Autodesk Inventor part; units mm, degrees
ref_plane "YZ Plane" through (0, 0, 0) normal (1, 0, 0) x (0, 1, 0)
ref_plane "XZ Plane" through (0, 0, 0) normal (0, 1, 0) x (-1, 0, 0)
ref_plane "XY Plane" through (0, 0, 0) normal (0, 0, 1) x (1, 0, 0)
sketch "Sketch1" plane through (0, 0, 0) normal (0, 0, 1) x (1, 0, 0)
  line L0 (100.1576, -44) -> (109, -35.1576)
  line L1 (109, -35.1576) -> (109, 35)
  line L2 (109, 35) -> (41.05, 35)
  line L3 (41.05, 35) -> (28, 30)
  line L4 (28, 30) -> (-28, 30)
  line L5 (-28, 30) -> (-30, 28)
  line L6 (-30, 28) -> (-30, -28)
  line L7 (-30, -28) -> (-28, -30)
  line L8 (-28, -30) -> (28, -30)
  line L9 (28, -30) -> (90.0667, -30)
  line L10 (90.0667, -30) -> (90.0667, -44)
  line L11 (90.0667, -44) -> (100.1576, -44)
  circle A0 centre (101, -8.23) radius 1.6
  circle A1 centre (101, 1.77) radius 1.6
  circle A2 centre (101, 29.77) radius 1.6
  circle A3 centre (85, 29.77) radius 1.6
  circle A4 centre (85, 1.77) radius 1.6
  circle A5 centre (85, -8.23) radius 1.6
  circle A6 centre (64.15, 11.27) radius 1.6
  circle A7 centre (47.85, 11.27) radius 1.6
  circle A8 centre (25, 0) radius 1.95
  circle A9 centre (0, 25) radius 1.95
  circle A10 centre (-25, -25) radius 1.95
  circle A11 centre (25, 25) radius 1.95
  circle A12 centre (-25, 25) radius 1.95
  circle A13 centre (25, -25) radius 1.95
  circle A14 centre (0, -25) radius 1.95
  circle A15 centre (-25, 0) radius 1.95
  circle A16 centre (-17.5, 17.5) radius 4
  circle A17 centre (17.5, -17.5) radius 4
  circle A18 centre (-17.5, -17.5) radius 4
  circle A19 centre (17.5, 17.5) radius 4
  line L12 (30, 28) -> (28, 30)
  line L13 (30, -28) -> (30, 28)
  line L14 (28, -30) -> (30, -28)
  point P0 (0, 0)
extrude "Extrusion1" add sketch "Sketch1" along normal blind 5 contours L8 L7 L6 L5 L4 L12 L13 L14
properties part number "cellSTORM_v5_spacer_xy_stage"
The listing builds one solid part. Answer for the finished solid, in the listing's coordinates (mm). Give positions to 0.01 mm unless a question says otherwise; leave off trailing zeros. Write each loop counter-clockwise with the first axis right and the second up, starting at its lowest first coordinate (ties: lowest second). Pieces come first, ordered by that corner, then holes. Notation, with made-up numbers: (-25, 69.25) -> (-20, 69.25) arc R17 ccw to (-20, 86.25) -> close; hole circle Ø9 at (51, 82.25). An arc over 180 degrees is marked (long way). Use a Markdown table: item, result.
(1) Section C-C, the plane x = 25 is taken. Determine the outline of the cut face in (y, z), then the cut area to 4 significant figures.
Return value:
| item | result |
|---|---|
| outline | (-30, 0) -> (-26.95, 0) -> (-26.95, 5) -> (-30, 5) -> close; (-23.05, 0) -> (-1.95, 0) -> (-1.95, 5) -> (-23.05, 5) -> close; (1.95, 0) -> (23.05, 0) -> (23.05, 5) -> (1.95, 5) -> close; (26.95, 0) -> (30, 0) -> (30, 5) -> (26.95, 5) -> close |
| area | 241.5 mm2 |
(2) Section A-A, the plane x = -17.5 is taken. Determine the outline of the cut face in (y, z), then the cut area to 3 significant figures.
Return value:
| item | result |
|---|---|
| outline | (-30, 0) -> (-21.5, 0) -> (-21.5, 5) -> (-30, 5) -> close; (-13.5, 0) -> (13.5, 0) -> (13.5, 5) -> (-13.5, 5) -> close; (21.5, 0) -> (30, 0) -> (30, 5) -> (21.5, 5) -> close |
| area | 220 mm2 |
(3) Determine the mould class of faces 1 (the cylindrical face through (23.052, -0.086, 2.465)), 2 (the flat face through (-30, 0, 2)), 3 (the flat face through (0, 0, 5)) for opening direction X: released by +X, released by -X, zero draft, split by the parting line, or undercut.
Return value:
| item | result |
|---|---|
| face 1 | undercut |
| face 2 | released by -X |
| face 3 | zero draft |
(4) Find the intervals of material crossed by probe 1 along Y at (x, z) = (-25, 1.85); probe 2 along Y at (x, z) = (-24, 0.75); probe 3 along X at (y, z) = (-16.5, 3.85), in increasing order. Write a range as from..to.
Return value:
| item | result |
|---|---|
| probe 1 | -30..-26.95, -23.05..-1.95, 1.95..23.05, 26.95..30 |
| probe 2 | -30..-26.67, -23.33..-1.67, 1.67..23.33, 26.67..30 |
| probe 3 | -30..-21.37, -13.63..13.63, 21.37..30 |
